The model under review builds one solid part; all positions refer to its coordinate system, in mm. Face numbers are marked on the shaded views. A direction names the side the tool comes from. Round coordinates to 2 decimals unless told otherwise and drop trailing zeros. Loops run counter-clockwise (first coordinate to the right, second up) from the corner with the lowest first, then second, coordinate; pieces in that order, holes last. Notation, with made-up numbers: M 29,86 L 85,86 A30 cw 85,122 Z; hole C 47.25,-1 d10. An arc over 180 degrees is marked long. Answer as a JSON object with one key per item and string values. Group by question number.
Item 1: Tool access review of the marked faces 1 and 2: name each direction out of +Z, -Z, +X, -X, +Y, -Y from which nothing blocks a thin tool from reaching the whole face with its end or side.
Item 2: Consider section B-B (y = -369). Give the boundary of the cut face in (x, z), and give its area (3 significant figures).
Item 3: Insertion check: P1, Ø1.5, axis at y = -80, z = 26.5, coming from the -X side; P2, Ø4, axis at x = -23.5, z = 7.5, coming from the -Y side; P3, Ø12, axis at y = -11, z = 23.5, coming from the +X side; P4, Ø1.5, axis at x = 9.5, y = -356, coming from the -Z side. Each pin has a flat end and moves straight along its axis. Give the tip position at first contact, or say it passes through.
Item 4: Consider section A-A (x = 0). Give the boundary of the cut face in (y, z).
Item 5: To check wall thickness, follow line 1 (Y direction, x = 45, z = 1.5); line 2 (X direction, y = -402, z = -23); line 3 (Z direction, x = 17.5, y = -172). State the ranges of each line that lie inside material, in increasing order.
```python
from build123d import *

# Parameters (mm, degrees)
BOSS_EXTRUDE1_DEPTH = 45
SKETCH3_R           = 25
BOSS_EXTRUDE2_DEPTH = 445
CHAMFER1_SIZE       = 4


with BuildPart() as part:
    # Sketch2 → Boss-Extrude1 (new body)
    with BuildSketch(Plane(origin=(0, 0, 0), x_dir=(1, 0, 0), z_dir=(0, 1, 0))):
        Polygon((80.829037687, 0), (40.414518843, 70), (-40.414518843, 70), (-80.829037687, 0), (-40.414518843, -70), (40.414518843, -70), align=None)
    extrude(amount=BOSS_EXTRUDE1_DEPTH)

    # Sketch3 → Boss-Extrude2 (add)
    with BuildSketch(Plane(origin=(0, 0, 0), x_dir=(1, 0, 0), z_dir=(0, 1, 0))):
        Circle(SKETCH3_R)
    extrude(amount=-BOSS_EXTRUDE2_DEPTH)

    # Sketch4 → Cut-Revolve1 (revolve, cut)
    with BuildSketch(Plane.XY):
        with BuildLine():
            Line((80.829037687, 33), (80.829037687, 45))
            Line((80.829037687, 45), (68.829037687, 45))
            ThreePointArc((68.829037687, 45), (77.314319061, 41.485281374), (80.829037687, 33))
        make_face()
    revolve(axis=Axis((0, 0, 0), (0, 1, 0)), mode=Mode.SUBTRACT)

    # Chamfer1
    chamfer1_edges = [part.edges().sort_by_distance(p)[0] for p in [
        (-25, -445, 0),
    ]]
    chamfer(chamfer1_edges, length=CHAMFER1_SIZE)


solid = part.part
```
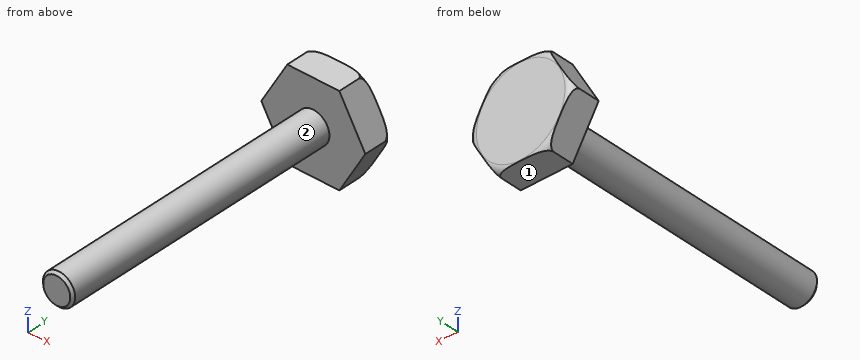
Geometry results:
{
 "1": {"face 1": "-Z, +X, -X, +Y, -Y", "face 2": "-Y"},
 "2": {"outline": "C 0,0 d50", "area": "1,960 mm^2"},
 "3": {"P1": "passes through", "P2": "stops at y = -443.33", "P3": "stops at x = 17.85", "P4": "stops at z = -23.42"},
 "4": {"outline": "M -445,-21 L -441,-25 L 0,-25 L 0,-70 L 44.94,-70 A12 ccw 45,-68.83 L 45,68.83 A12 ccw 44.94,70 L 0,70 L 0,25 L -441,25 L -445,21 Z"},
 "5": {"line 1": "y = 0 to 45", "line 2": "x = -9.8 to 9.8", "line 3": "z = -17.85 to 17.85"}
}
